```python
from build123d import *

# Parameters (mm, degrees)
F0_W     = 9.0247368789
F0_H     = 5.08
F0_W_2   = 5.08
F0_H_2   = 4.9726772237
F0_W_3   = 7.5355667663
F0_H_3   = 4.96
F0_H_4   = 4.9763912218
F1_DEPTH = 2
F2_DEPTH = 4
F4_D     = 3
F4_DEPTH = 3
F4_TIP   = 0.9012909285
F0_W_4   = 2
F0_H_5   = 19.347961992
F5_DEPTH = 30
F0_H_6   = 9.4683412462
F0_H_7   = 12.5924479216
F0_W_5   = 9.5816506073
F0_H_8   = 2
F0_H_9   = 53.2766682494
F6_DEPTH = 5


with BuildPart() as f1:
    # F0 (on Top) → F1 (new body)
    with BuildSketch(Plane.XY):
        Polygon((12.5546930358, 21.8509457558), (-55.8220994771, 21.8509457558), (-55.8220994771, 12.5924479216), (-55.8220994771, 0), (-55.8220994771, -19.347961992), (-55.8220994771, -28.8163032383), (-55.8220994771, -32.4290542442), (38.6587072041, -32.4290542442), (38.6587072041, -31.9290542442), (38.6587072041, 21.3476140052), (38.6587072041, 21.8509457558), (22.1363436431, 21.8509457558), align=None)
        with Locations((-41.3520994771, -29.3890542442)):
            Rectangle(F0_W, F0_H, mode=Mode.SUBTRACT)
        with Locations((10.7179005229, -24.3090542442)):
            Rectangle(F0_W_2, F0_H_2, mode=Mode.SUBTRACT)
        with Locations((-40.0820994771, 18.8709457558)):
            Rectangle(F0_W_3, F0_H_3, mode=Mode.SUBTRACT)
        with Locations((10.7179005229, 3.6309457558)):
            Rectangle(F0_W_2, F0_H_4, mode=Mode.SUBTRACT)
    extrude(amount=F1_DEPTH)

    # F0 (on Top) → F2 (join)
    with BuildSketch(Plane.XY):
        with Locations((-40.0820994771, 18.8709457558)):
            Rectangle(F0_W_3, F0_H_3)
        with Locations((10.7179005229, 3.6309457558)):
            Rectangle(F0_W_2, F0_H_4)
        with Locations((10.7179005229, -24.3090542442)):
            Rectangle(F0_W_2, F0_H_2)
        with Locations((-41.3520994771, -29.3890542442)):
            Rectangle(F0_W, F0_H)
    extrude(amount=F2_DEPTH)

    # F4
    with Locations(Plane.XY.offset(4)):
        with Locations((-40.0820994771, 18.8709457558), (-41.3520994771, -29.3890542442), (10.7179005229, -24.3090542442), (10.7179005229, 3.6309457558)):
            Hole(F4_D / 2, depth=F4_DEPTH)
            with Locations((0, 0, -(F4_DEPTH + F4_TIP / 2))):  # 118° drill point
                Cone(0, F4_D / 2, F4_TIP, mode=Mode.SUBTRACT)

    # F0 (on Top) → F5 (join)
    with BuildSketch(Plane.XY):
        Polygon((-55.8220994771, -32.4290542442), (-55.8220994771, -28.8163032383), (-57.8220994771, -28.8163032383), (-57.8220994771, -34.4290542442), (40.6587072041, -34.4290542442), (40.6587072041, -31.9290542442), (38.6587072041, -31.9290542442), (38.6587072041, -32.4290542442), align=None)
        Polygon((-55.8220994771, 12.5924479216), (-55.8220994771, 21.8509457558), (12.5546930358, 21.8509457558), (12.5546930358, 23.8509457558), (-57.8220994771, 23.8509457558), (-57.8220994771, 12.5924479216), align=None)
        with Locations((-56.8220994771, -9.673980996)):
            Rectangle(F0_W_4, F0_H_5)
        Polygon((22.1363436431, 23.8509457558), (22.1363436431, 21.8509457558), (38.6587072041, 21.8509457558), (38.6587072041, 21.3476140052), (40.6587072041, 21.3476140052), (40.6587072041, 23.8509457558), align=None)
    extrude(amount=F5_DEPTH)

    # F0 (on Top) → F6 (join)
    with BuildSketch(Plane.XY):
        with Locations((-56.8220994771, -24.0821326151)):
            Rectangle(F0_W_4, F0_H_6)
        with Locations((-56.8220994771, 6.2962239608)):
            Rectangle(F0_W_4, F0_H_7)
        with Locations((17.3455183394, 22.8509457558)):
            Rectangle(F0_W_5, F0_H_8)
        with Locations((39.6587072041, -5.2907201195)):
            Rectangle(F0_W_4, F0_H_9)
    extrude(amount=F6_DEPTH)


solid = f1.part
```
Part model, mm, in its own coordinate system. A direction names the side the tool comes from. Coordinates: 2 decimals unless noted, no trailing zeros. Order: outer loops, then holes, each group sorted by start corner. A loop starts at its lowest first (then second) coordinate and runs counter-clockwise, first axis right, second up. Notation, with made-up numbers: (-20.5, 82.25) -> (14.5, 82.25) arc R18 cw to (14.5, 113.25) -> close; hole circle Ø6 at (87.25, -35.75). An arc over 180 degrees is marked (long way). Put each result on its own line as item: value. Start each with the question number.
(1) Pin check, flat tips, straight feed: pin 1 Ø1.5 at (x, y) = (0, -9) entering from +Z; pin 2 Ø0.6 at (x, y) = (40, -4) entering from +Z. Stop position of each tip, or through.
(2) Which spindle directions (+Z, -Z, +X, -X, +Y, -Y) get a long thin tool onto all of the face, cutting with end or side? Do faces 4 (the face through (12.555, 23, 17)), 5 (the face through (-36.84, -29, 3)), 6 (the face through (-57, 12.592, 17)), 7 (the face through (31, 23, 30)). Say none if no direction does.
(3) Band-saw the part on A-A (z = 10.5). Give the cut face in (x, y).
(4) Band-saw the part on C-C (x = 29). Give the cut face in (y, z), then the cut area to 3 significant figures.
(5) Probe line 1 along Y through (x, z) = (-35, 16.75); line 2 along X through (y, z) = (8, 4.75); line 3 along X through (y, z) = (-30, 6). List the from-to ranges inside material, lowest first. Write a range as [from, to].
(6) Mould opens along Y. For faces 1 (the face through (-8, 23.851, 15)), 2 (the face through (-57, -10, 30)), 3 (the face through (12, -23, 4)) say: pulls with the +Y half, pulls with the -Y half, needs draft (parallel to the pull), parting line crosses it, or undercut.
(7) Band-saw the part on B-B (y = -15). Give the cut face in (x, z).
Determined:
1. pin 1: stops at z = 2
1. pin 2: stops at z = 5
2. face 4: +Z, +Y
2. face 5: +Z
2. face 6: +Z, +X, -X
2. face 7: +Z, +X, -X, +Y, -Y
3. outline: (-57.82, -34.43) -> (40.66, -34.43) -> (40.66, -31.93) -> (38.66, -31.93) -> (38.66, -32.43) -> (-55.82, -32.43) -> (-55.82, -28.82) -> (-57.82, -28.82) -> close; (-57.82, -19.35) -> (-55.82, -19.35) -> (-55.82, 0) -> (-57.82, 0) -> close; (-57.82, 12.59) -> (-55.82, 12.59) -> (-55.82, 21.85) -> (12.55, 21.85) -> (12.55, 23.85) -> (-57.82, 23.85) -> close; (22.14, 21.85) -> (38.66, 21.85) -> (38.66, 21.35) -> (40.66, 21.35) -> (40.66, 23.85) -> (22.14, 23.85) -> close
4. outline: (-34.43, 0) -> (23.85, 0) -> (23.85, 30) -> (21.85, 30) -> (21.85, 2) -> (-32.43, 2) -> (-32.43, 30) -> (-34.43, 30) -> close
4. area: 229 mm²
5. line 1: y = [-34.43, -32.43], [21.85, 23.85]
5. line 2: x = [-57.82, -55.82], [38.66, 40.66]
5. line 3: x = [-57.82, -55.82]
6. face 1: pulls with the +Y half
6. face 2: needs draft
6. face 3: undercut
7. outline: (-57.82, 0) -> (40.66, 0) -> (40.66, 5) -> (38.66, 5) -> (38.66, 2) -> (-55.82, 2) -> (-55.82, 30) -> (-57.82, 30) -> close
